from build123d import *

# Parameters (mm, degrees)
SKETCH1_R                   = 4
SKETCH1_R_2                 = 3
EXTRUDE_THIN1_DEPTH         = 215.5
SKETCH3_W                   = 1.25
SKETCH3_H                   = 5.465467641
M3_TAPPED_HOLE1_AT_2_COUNT  = 2
M3_TAPPED_HOLE1_AT_2_PITCH  = 11
CIRPATTERN1_COUNT           = 3
CIRPATTERN1_COPY_1_SKETCH_W = 1.25
CIRPATTERN1_COPY_1_SKETCH_H = 5.465467641
CIRPATTERN1_COPY_2_SKETCH_W = 1.25
CIRPATTERN1_COPY_2_SKETCH_H = 5.465467641


with BuildPart() as part:
    # Sketch1 → Extrude-Thin1 (new, symmetric)
    with BuildSketch(Plane(origin=(0, 0, 0), x_dir=(0, 0, -1), z_dir=(1, 0, 0))):
        Circle(SKETCH1_R)
        Circle(SKETCH1_R_2, mode=Mode.SUBTRACT)
    extrude(amount=EXTRUDE_THIN1_DEPTH, both=True)

    # Sketch3 → M3 Tapped Hole1 (revolve, cut)
    with BuildSketch(Plane(origin=(-5.5, 0, 0), x_dir=(0, 0, -1), z_dir=(1, 0, 0))):
        with Locations((0.625, 2.732733821)):
            Rectangle(SKETCH3_W, SKETCH3_H)
    m3_tapped_hole1 = revolve(axis=Axis((-5.5, -6.35, 0), (0, 1, 0)), mode=Mode.SUBTRACT)

    # M3 Tapped Hole1 at 2: M3 Tapped Hole1 ×2
    with Locations(*[(i * M3_TAPPED_HOLE1_AT_2_PITCH, 0, 0) for i in range(1, M3_TAPPED_HOLE1_AT_2_COUNT)]):
        add(m3_tapped_hole1, mode=Mode.SUBTRACT)

    # CirPattern1: M3 Tapped Hole1 ×3 about axis
    cirpattern1_axis = Axis((215.5, 0, 0), (-1, 0, 0))
    for i in range(1, CIRPATTERN1_COUNT):
        add(m3_tapped_hole1.rotate(cirpattern1_axis, i * 360 / CIRPATTERN1_COUNT), mode=Mode.SUBTRACT)

    # CirPattern1 copy 1 sketch → CirPattern1 copy 1 (revolve, cut)
    with BuildSketch(Plane(origin=(5.5, 0, 0), x_dir=(0, -0.8660254037844387, 0.4999999999999998), z_dir=(1, 0, 0))):
        with Locations((0.625, 2.732733821)):
            Rectangle(CIRPATTERN1_COPY_1_SKETCH_W, CIRPATTERN1_COPY_1_SKETCH_H)
    revolve(axis=Axis((5.5, 3.175, 5.499261314), (0, -0.4999999999999998, -0.8660254037844387)), mode=Mode.SUBTRACT)

    # CirPattern1 copy 2 sketch → CirPattern1 copy 2 (revolve, cut)
    with BuildSketch(Plane(origin=(5.5, 0, 0), x_dir=(0, 0.8660254037844384, 0.5000000000000004), z_dir=(1, 0, 0))):
        with Locations((0.625, 2.732733821)):
            Rectangle(CIRPATTERN1_COPY_2_SKETCH_W, CIRPATTERN1_COPY_2_SKETCH_H)
    revolve(axis=Axis((5.5, 3.175, -5.499261314), (0, -0.5000000000000004, 0.8660254037844384)), mode=Mode.SUBTRACT)


solid = part.part
Verification items for the finished model (mm, model axes). Give positions to 0.01 mm unless a question says otherwise; leave off trailing zeros. Loops run counter-clockwise (first coordinate to the right, second up) from the corner with the lowest first, then second, coordinate; pieces in that order, holes last.
1. Material ranges on probe 1 along X at (y, z) = (3.4, 0); probe 2 along Y at (x, z) = (143, -0.5); probe 3 along X at (y, z) = (-2.5, -3), recorded low to high.
Derived:
probe 1: x = -215.5 to -6.75, -4.25 to 4.25, 6.75 to 215.5
probe 2: y = -3.97 to -2.96, 2.96 to 3.97
probe 3: x = -215.5 to -6.56, -4.44 to 4.44, 6.56 to 215.5
2. Go/stop test with flat-tipped pins: P1, Ø4, axis at x = -137.5, z = -2.5, coming from the +Y side; P2, Ø2, axis at x = -22.5, z = -3, coming from the +Y side. Record where each tip stops, or that it passes through.
Derived:
P1: stops at y = 3.97
P2: stops at y = 3.46
3. Cross-section at B-B on x = -66.5. Record the cut outline in (y, z).
Derived:
outline: circle Ø8 at (0, 0); hole circle Ø6 at (0, 0)
4. Cross-section at A-A on z = 0. Record the cut outline in (x, y).
Derived:
outline: (-215.5, -4) - (215.5, -4) - (215.5, -3) - (-215.5, -3) - close; (-215.5, 3) - (-6.75, 3) - (-6.75, 4) - (-215.5, 4) - close; (-4.25, 3) - (4.25, 3) - (4.25, 4) - (-4.25, 4) - close; (6.75, 3) - (215.5, 3) - (215.5, 4) - (6.75, 4) - close
